Geometry check sheet. Reference: the model listing, model coordinates, mm. A direction names the side the tool comes from. Round coordinates to 2 decimals unless told otherwise and drop trailing zeros. Write each loop counter-clockwise with the first axis right and the second up, starting at its lowest first coordinate (ties: lowest second). Pieces come first, ordered by that corner, then holes.
Item 1: Cross-section at B-B (z = 26). Enter the section's corners in (x, y), then the cut area to 3 significant figures.
Item 2: Access from +Z, -Z, +X, -X, +Y, -Y to the whole of each face (thin tool, end or side, straight path). Record for faces 4 (the face through (12, 32, 9)), 5 (the face through (-38, 8, 1.957)), 6 (the face through (-19, 24, 18.043)), 7 (the face through (-4, 44, 9)), 8 (the face through (-48, 8, 16)).
Item 3: Cross-section at C-C (x = -1.5). Enter the section's corners in (y, z).
Item 4: Cross-section at A-A (y = 12). Enter the section's corners in (x, z).
Item 5: Draft check along Z on faces 1 (the face through (-38, 8, -14.043)), 2 (the face through (10, 18, 30.043)), 3 (the face through (28, 44, 9)). Enter one of: pulls with the +Z half, pulls with the -Z half, needs draft (parallel to the pull), parting line crosses it, or undercut.
Item 6: Scan lines: probe 1 along Z at (x, y) = (22, 36); probe 2 along Y at (x, z) = (-4.5, -19); probe 3 along Y at (x, z) = (24.5, -4.5). Record each from-to range of solid material in increasing order.
Item 7: Cross-section at D-D (y = 24.5). Enter the section's corners in (x, z).
Item 8: Depth check by flat-ended pin: P1, Ø12, axis at y = 41, z = -4.5, coming from the -X side; P2, Ø14, axis at x = 9, y = 30, coming from the -Z side; P3, Ø8, axis at x = -18, y = 43, coming from the +Z side; P4, Ø10, axis at x = -18, y = 32, coming from the -Z side. Enter the tip coordinate at first touch or a pass-through.
from build123d import *

# Parameters (mm, degrees)
SKETCH1_W           = 96
SKETCH1_H           = 60.085106382
BOSS_EXTRUDE2_DEPTH = 16
BOSS_EXTRUDE3_DEPTH = 16
SKETCH5_W           = 40
SKETCH5_H           = 42
BOSS_EXTRUDE4_DEPTH = 28
SKETCH6_R           = 12
CUT_EXTRUDE1_DEPTH  = 43
BOSS_EXTRUDE6_DEPTH = 12
CUT_EXTRUDE2_DEPTH  = 16


with BuildPart() as part:
    # Sketch1 → Boss-Extrude2 (new body)
    with BuildSketch(Plane(origin=(0, 0, 0), x_dir=(1, 0, 0), z_dir=(0, 1, 0))):
        Rectangle(SKETCH1_W, SKETCH1_H)
    extrude(amount=BOSS_EXTRUDE2_DEPTH)

    # Sketch4 → Boss-Extrude3 (add)
    with BuildSketch(Plane(origin=(48, 0, 0), x_dir=(0, 0, -1), z_dir=(1, 0, 0))):
        with BuildLine():
            Line((-30.042553191, 16), (-30.042553191, 64))
            ThreePointArc((-30.042553191, 64), (12.027119449, 55.055223992), (30.042553191, 16))
            Line((30.042553191, 16), (30.042553191, 0))
            Line((30.042553191, 0), (-30.042553191, 0))
            Line((-30.042553191, 0), (-30.042553191, 16))
        make_face()
    extrude(amount=-BOSS_EXTRUDE3_DEPTH)

    # Sketch5 → Boss-Extrude4 (add)
    with BuildSketch(Plane(origin=(0, 16, 0), x_dir=(1, 0, 0), z_dir=(0, 1, 0))):
        with Locations((12, -9.042553191)):
            Rectangle(SKETCH5_W, SKETCH5_H)
    extrude(amount=BOSS_EXTRUDE4_DEPTH)

    # Sketch6 → Cut-Extrude1 (cut)
    with BuildSketch(Plane.XY.offset(30.042553191)):
        with Locations((12, 44)):
            Circle(SKETCH6_R)
    extrude(amount=-CUT_EXTRUDE1_DEPTH, mode=Mode.SUBTRACT)

    # Sketch10 → Boss-Extrude6 (add)
    with BuildSketch(Plane.XY.offset(30.042553191)):
        Polygon((-8, 44), (-48, 16), (-8, 16), align=None)
    extrude(amount=-BOSS_EXTRUDE6_DEPTH)

    # Sketch11 → Cut-Extrude2 (cut)
    with BuildSketch(Plane(origin=(0, 16, 0), x_dir=(1, 0, 0), z_dir=(0, 1, 0))):
        with BuildLine():
            Line((-28, 14.042553191), (-48, 14.042553191))
            Line((-48, 14.042553191), (-48, -1.957446809))
            Line((-48, -1.957446809), (-28, -1.957446809))
            ThreePointArc((-28, -1.957446809), (-36, 6.042553191), (-28, 14.042553191))
        make_face()
        with BuildLine():
            ThreePointArc((-20, 6.042553191), (-22.343145751, 11.699407441), (-28, 14.042553191))
            Line((-28, 14.042553191), (-28, -1.957446809))
            ThreePointArc((-28, -1.957446809), (-22.343145751, 0.385698942), (-20, 6.042553191))
        make_face()
        with BuildLine():
            Line((-28, -1.957446809), (-28, 14.042553191))
            ThreePointArc((-28, 14.042553191), (-36, 6.042553191), (-28, -1.957446809))
        make_face()
    extrude(amount=-CUT_EXTRUDE2_DEPTH, mode=Mode.SUBTRACT)


solid = part.part
Resolved:
1. outline: (-48, 0) - (48, 0) - (48, 64.87) - (32, 64.87) - (32, 44) - (24, 44) arc R12 cw to (0, 44) - (-8, 44) - (-48, 16) - close
1. area: 3,770 mm2
2. face 4: +Z, -Z, +Y
2. face 5: -X, +Y, -Y
2. face 6: -Z, -X, +Y
2. face 7: +Z, -Z, -X, +Y
2. face 8: +Z, -Z, -X, +Y, -Y
3. outline: (0, -30.04) - (16, -30.04) - (16, -11.96) - (44, -11.96) - (44, 30.04) - (0, 30.04) - close
4. outline: (-48, -30.04) - (48, -30.04) - (48, 30.04) - (-48, 30.04) - (-48, 1.96) - (-28, 1.96) arc R8 cw to (-28, -14.04) - (-48, -14.04) - close
5. face 1: undercut
5. face 2: pulls with the +Z half
5. face 3: needs draft
6. probe 1: z = -11.96 to 30.04
6. probe 2: y = 0 to 16
6. probe 3: y = 0 to 44
7. outline: (-35.86, 18.04) - (-8, 18.04) - (-8, -11.96) - (32, -11.96) - (32, -29.56) - (48, -29.56) - (48, 30.04) - (-35.86, 30.04) - close
8. P1: stops at x = -8
8. P2: stops at z = -11.96
8. P3: passes through
8. P4: stops at z = 18.04
